```python
from build123d import *

# Parameters (mm, degrees)
SKETCH1_R           = 15.988284
BOSS_EXTRUDE1_DEPTH = 3.175
SKETCH2_R           = 30.48
CUT_EXTRUDE1_DEPTH  = 4.175
SKETCH4_R           = 1.499997
SKETCH4_R_2         = 3.2004
CUT_EXTRUDE2_DEPTH  = 4.175


with BuildPart() as part:
    # Sketch1 → Boss-Extrude1 (new body)
    with BuildSketch(Plane(origin=(0, 0, 0), x_dir=(1, 0, 0), z_dir=(0, 1, 0))):
        Circle(SKETCH1_R)
    extrude(amount=BOSS_EXTRUDE1_DEPTH)

    # Sketch2 → Cut-Extrude1 (cut, through all)
    with BuildSketch(Plane(origin=(0, 3.175, 0), x_dir=(1, 0, 0), z_dir=(0, 1, 0))):
        with Locations((-35.938985022, 0)):
            Circle(SKETCH2_R)
    extrude(amount=-CUT_EXTRUDE1_DEPTH, mode=Mode.SUBTRACT)

    # Sketch4 → Cut-Extrude2 (cut, through all)
    with BuildSketch(Plane(origin=(0, 3.175, 0), x_dir=(1, 0, 0), z_dir=(0, 1, 0))):
        with Locations((0, 7.999984)):
            Circle(SKETCH4_R)
        with Locations((0, -7.999984)):
            Circle(SKETCH4_R)
        with Locations((7.999984, 0)):
            Circle(SKETCH4_R)
        Circle(SKETCH4_R_2)
    extrude(amount=-CUT_EXTRUDE2_DEPTH, mode=Mode.SUBTRACT)


solid = part.part
```
Work out the finished part from the listing and answer in its coordinate system (mm). Round coordinates to 2 decimals unless told otherwise and drop trailing zeros. Write each loop counter-clockwise with the first axis right and the second up, starting at its lowest first coordinate (ties: lowest second). Pieces come first, ordered by that corner, then holes. Notation, with made-up numbers: (82.25, 62.5) - (109.25, 62.5) arc R18 ccw to (109.25, 92.5) - close; hole circle Ø7 at (-25, -8). An arc over 180 degrees is marked (long way). Return JSON: item names as keys, results as strings. Group by question number.
Q1. This flat-tipped pin is pushed along its axis until it touches: pin 1 Ø1.5 at (x, y) = (-3.5, 1) entering from +Z. Where does it stop, or does it pass through?
Q2. The part is cut by section B-B on x = 0. Write down the section's boundary in (y, z) (3 decimals), then the cut area to 3 significant figures.
Q3. The part is cut by section C-C on x = -2.5. Write down the section's boundary in (y, z) (3 decimals), then the cut area to 3 significant figures.
Q4. The part is cut by section A-A on z = 0. Write down the section's boundary in (x, y) (3 decimals), then the cut area to 3 significant figures.
Q5. Find the intervals of material crossed by L1, parallel to Z at x = 0, y = 0.8; L2, parallel to X at y = 2.05, z = 0; L3, parallel to Z at x = 2.25, y = 2.15, in increasing order.
Q6. The part is cut by section D-D on y = 2.65. Write down the section's boundary in (x, z), then the cut area to 3 significant figures.
Solved:
{
 "1": {"pin 1": "z = 15.75"},
 "2": {"outline": "(0, -15.988) - (3.175, -15.988) - (3.175, -9.5) - (0, -9.5) - close; (0, -6.5) - (3.175, -6.5) - (3.175, -3.2) - (0, -3.2) - close; (0, 3.2) - (3.175, 3.2) - (3.175, 6.5) - (0, 6.5) - close; (0, 9.5) - (3.175, 9.5) - (3.175, 15.988) - (0, 15.988) - close", "area": "62.2 mm²"},
 "3": {"outline": "(0, -15.792) - (3.175, -15.792) - (3.175, -1.998) - (0, -1.998) - close; (0, 1.998) - (3.175, 1.998) - (3.175, 15.792) - (0, 15.792) - close", "area": "87.6 mm²"},
 "4": {"outline": "(-5.459, 0) - (-3.2, 0) - (-3.2, 3.175) - (-5.459, 3.175) - close; (3.2, 0) - (6.5, 0) - (6.5, 3.175) - (3.2, 3.175) - close; (9.5, 0) - (15.988, 0) - (15.988, 3.175) - (9.5, 3.175) - close", "area": "38.2 mm²"},
 "5": {"L1": "-15.99 to -9.5, -6.5 to -3.2, 3.2 to 6.5, 9.5 to 15.99", "L2": "-5.46 to -3.2, 3.2 to 6.5, 9.5 to 15.99", "L3": "-15.83 to -2.28, 2.28 to 15.83"},
 "6": {"outline": "(-8.6, -13.48) arc R15.99 ccw (long way) to (-8.6, 13.48) arc R30.48 cw to start; hole circle Ø6.4 at (0, 0); hole circle Ø3 at (0, -8); hole circle Ø3 at (0, 8); hole circle Ø3 at (8, 0)", "area": "552 mm²"}
}
